```python
from build123d import *

# Parameters (mm, degrees)
SKETCH_1_W                    = 17
SKETCH_1_H                    = 45
EXTRUDE_293_DEPTH             = 10
HOLE_WIZARD_40_M5_D           = 5.5
HOLE_WIZARD_40_M5_CSINK_D     = 10.4
HOLE_WIZARD_40_M5_CSINK_ANGLE = 90
HOLE_WIZARD_1122_D            = 2.5
HOLE_WIZARD_1122_CSINK_D      = 3.05
HOLE_WIZARD_1122_CSINK_ANGLE  = 90
CHAMFER_1_SIZE                = 0.5


with BuildPart() as part:
    # Эскиз1 → Extrude 293 (new body)
    with BuildSketch(Plane(origin=(0, 0, 0), x_dir=(1, 0, 0), z_dir=(0, 1, 0))):
        Rectangle(SKETCH_1_W, SKETCH_1_H)
    extrude(amount=EXTRUDE_293_DEPTH)

    # Крепление к профилю 40 - M5 (through all)
    with Locations(Plane(origin=(0, 10, 0), x_dir=(-1, 0, 0), z_dir=(0, 1, 0))):
        with Locations((0, 0)):
            CounterSinkHole(HOLE_WIZARD_40_M5_D / 2, HOLE_WIZARD_40_M5_CSINK_D / 2, counter_sink_angle=HOLE_WIZARD_40_M5_CSINK_ANGLE)

    # Hole Wizard 1122 (through all)
    with Locations(Plane(origin=(0, 10, 0), x_dir=(-1, 0, 0), z_dir=(0, 1, 0))):
        with Locations((5.55, 8.95), (-5.55, 8.95)):
            CounterSinkHole(HOLE_WIZARD_1122_D / 2, HOLE_WIZARD_1122_CSINK_D / 2, counter_sink_angle=HOLE_WIZARD_1122_CSINK_ANGLE)

    # Фаска1
    chamfer_1_edges = [part.edges().sort_by_distance(p)[0] for p in [
        (-8.5, 10, 0),
        (8.5, 10, 0),
        (0, 10, -22.5),
    ]]
    chamfer(chamfer_1_edges, length=CHAMFER_1_SIZE)


solid = part.part
```
Model file for the job. Use its own axes, mm. Round coordinates to 2 decimals unless told otherwise and drop trailing zeros. Order: outer loops, then holes, each group sorted by start corner. A loop starts at its lowest first (then second) coordinate and runs counter-clockwise, first axis right, second up. Notation, with made-up numbers: (7.25, 52.5) -> (25.25, 52.5) arc R18 cw to (25.25, 60.5) -> close; hole circle Ø9 at (5.25, 77.5). An arc over 180 degrees is marked (long way). Use one line per item in the form item = value.
Item 1: Cut at A-A, the plane z = 0. Write the cut outline in (x, y).
Returned:
outline = (-8.5, 0) -> (-2.75, 0) -> (-2.75, 7.55) -> (-5.2, 10) -> (-8, 10) -> (-8.5, 9.5) -> close; (2.75, 0) -> (8.5, 0) -> (8.5, 9.5) -> (8, 10) -> (5.2, 10) -> (2.75, 7.55) -> close
Item 2: Cut at D-D, the plane z = 8.95. Write the cut outline in (x, y) (3 decimals), and give its area (3 significant figures).
Returned:
outline = (-8.5, 0) -> (-6.8, 0) -> (-6.8, 9.725) -> (-7.075, 10) -> (-8, 10) -> (-8.5, 9.5) -> close; (-4.3, 0) -> (4.3, 0) -> (4.3, 9.725) -> (4.025, 10) -> (-4.025, 10) -> (-4.3, 9.725) -> close; (6.8, 0) -> (8.5, 0) -> (8.5, 9.5) -> (8, 10) -> (7.075, 10) -> (6.8, 9.725) -> close
area = 120 mm^2
Item 3: Cut at B-B, the plane y = 1.5. Write the cut outline in (x, z), and give its area (3 significant figures).
Returned:
outline = (-8.5, -22.5) -> (8.5, -22.5) -> (8.5, 22.5) -> (-8.5, 22.5) -> close; hole circle Ø2.5 at (-5.55, 8.95); hole circle Ø5.5 at (0, 0); hole circle Ø2.5 at (5.55, 8.95)
area = 731 mm^2
Item 4: Cut at C-C, the plane x = 0. Write the cut outline in (y, z), and give its area (3 significant figures).
Returned:
outline = (0, -22.5) -> (9.5, -22.5) -> (10, -22) -> (10, -5.2) -> (7.55, -2.75) -> (0, -2.75) -> close; (0, 2.75) -> (7.55, 2.75) -> (10, 5.2) -> (10, 22.5) -> (0, 22.5) -> close
area = 389 mm^2
Item 5: Pull direction Z, two halves, no side cores. Call faces 1 (the face through (8.5, 5, 0)), 2 (the face through (6.222, 4.794, 10.004)), 3 (the face through (0, 5, 22.5)): released by +Z, released by -Z, zero draft, split by the parting line, or undercut.
Returned:
face_1 = zero draft
face_2 = undercut
face_3 = released by +Z
Item 6: Flat gauge pins, fed straight in: pin 1 Ø9 at (x, z) = (0, 0) entering from +Y; pin 2 Ø3 at (x, z) = (-5.55, 8.95) entering from +Y (3 decimals). Where does each tip first touch, or does it go through?
Returned:
pin_1 = 9.3
pin_2 = 9.975
Item 7: Drill centre lines: line 1 (X direction, y = 5, z = 8.95); line 2 (Z direction, x = 5.55, y = 4.75); line 3 (Z direction, x = 0, y = 4.75). Where is each one in solid material? Low to high.
Returned:
line_1 = -8.5 to -6.8, -4.3 to 4.3, 6.8 to 8.5
line_2 = -22.5 to 7.7, 10.2 to 22.5
line_3 = -22.5 to -2.75, 2.75 to 22.5
